Part model, mm, in its own coordinate system. A direction names the side the tool comes from. Give positions to 0.01 mm unless a question says otherwise; leave off trailing zeros. Write each loop counter-clockwise with the first axis right and the second up, starting at its lowest first coordinate (ties: lowest second). Pieces come first, ordered by that corner, then holes.
```python
from build123d import *

# Parameters (mm, degrees)
SKETCH1_R           = 25
SKETCH1_R_2         = 0.9
BOSS_EXTRUDE1_DEPTH = 1.5875
CUT_EXTRUDE1_REACH  = 37.498
SKETCH2_W           = 3.873993702
SKETCH2_H           = 19.044786736


with BuildPart() as part:
    # Sketch1 → Boss-Extrude1 (new, symmetric)
    with BuildSketch(Plane.XY):
        Circle(SKETCH1_R)
        Circle(SKETCH1_R_2, mode=Mode.SUBTRACT)
    extrude(amount=BOSS_EXTRUDE1_DEPTH, both=True)

    # Sketch2 → Cut-Extrude1 (cut, up to next)
    with BuildSketch(Plane(origin=(0, 0, -1.5875), x_dir=(-1, 0, 0), z_dir=(0, 0, -1)), mode=Mode.PRIVATE) as cut_extrude1_sk1:
        with Locations((0, 24.522393368)):
            Rectangle(SKETCH2_W, SKETCH2_H)
    cut_extrude1_tool1 = extrude(cut_extrude1_sk1.sketch, amount=-CUT_EXTRUDE1_REACH, mode=Mode.PRIVATE) & part.part
    add(cut_extrude1_tool1.solids().sort_by_distance((0, 24.522393, -1.5875))[0], mode=Mode.SUBTRACT)


solid = part.part
```
1) Wall check: L1, parallel to Y at x = 0, z = 0.45; L2, parallel to Y at x = -4, z = 1.15; L3, parallel to Y at x = 14, z = 1.1. Give the ranges that are in metal, low to high.
Answers follow:
L1: y = -25 to -0.9, 0.9 to 15
L2: y = -24.68 to 24.68
L3: y = -20.71 to 20.71
2) Pin check, flat tips, straight feed: pin 1 Ø1 at (y, z) = (22, 0.5) entering from +X; pin 2 Ø1 at (y, z) = (15.5, -1) entering from +X; pin 3 Ø1.4 at (x, y) = (0, 0) entering from +Z; pin 4 Ø1 at (y, z) = (20, -0.5) entering from -X. Stop position of each tip, or through.
Answers follow:
pin 1: stops at x = 12.76
pin 2: stops at x = 20
pin 3: passes through
pin 4: stops at x = -15.64
3) Saw through at A-A, the plane y = 0. Write the cut outline in (x, z), then the cut area to 3 significant figures.
Answers follow:
outline: (-25, -1.59) - (-0.9, -1.59) - (-0.9, 1.59) - (-25, 1.59) - close; (0.9, -1.59) - (25, -1.59) - (25, 1.59) - (0.9, 1.59) - close
area: 153 mm2
4) Saw through at D-D, the plane y = 10.5. Write the cut outline in (x, z).
Answers follow:
outline: (-22.69, -1.59) - (22.69, -1.59) - (22.69, 1.59) - (-22.69, 1.59) - close
5) 3-axis set-ups, long thin cutter, end or side, ignore diameter. For faces 5 (the face through (0, -5, 1.588)), 6 (the face through (-1.937, 20, 0)): which of +Z, -Z, +X, -X, +Y, -Y reach the whole face in a straight line?
Answers follow:
face 5: +Z, +X, -X, +Y, -Y
face 6: +Z, -Z, +Y
6) Saw through at B-B, the plane x = 0. Write the cut outline in (y, z), then the cut area to 3 significant figures.
Answers follow:
outline: (-25, -1.59) - (-0.9, -1.59) - (-0.9, 1.59) - (-25, 1.59) - close; (0.9, -1.59) - (15, -1.59) - (15, 1.59) - (0.9, 1.59) - close
area: 121 mm2
7) Two-plate mould, pull along X, no slides. Class faces 1 (the face through (-1.072, -24.977, 0.022)), 2 (the face through (0, -5, -1.588)), 3 (the face through (0.86, 0.27, -0.02)), 4 (the face through (1.937, 20, 0)): +X half, -X half, draft (parallel to the pull), parting line (faces both ways), or undercut.
Answers follow:
face 1: parting line
face 2: draft
face 3: undercut
face 4: undercut
8) Saw through at C-C, the plane z = 1.05. Write the cut outline in (x, y), then the cut area to 3 significant figures.
Answers follow:
outline: (-1.94, 15) - (-1.94, 24.92) arc R25 ccw (long way) to (1.94, 24.92) - (1.94, 15) - close; hole circle Ø1.8 at (0, 0)
area: 1,920 mm2
